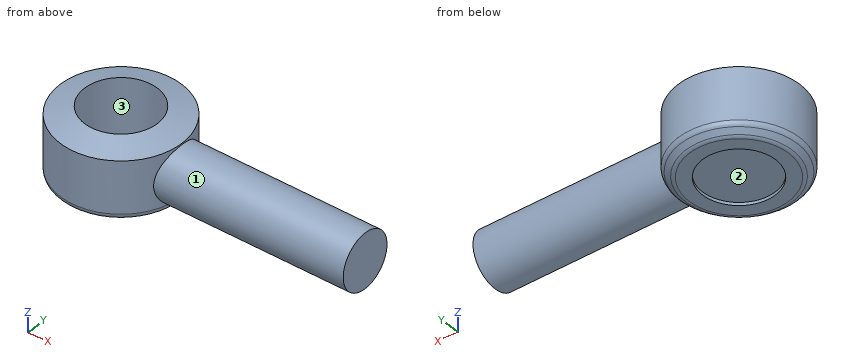
```python
from build123d import *

# Parameters (mm, degrees)
BOSS_EXTRUDE3_OUTLINE_W = 9
BOSS_EXTRUDE3_OUTLINE_H = 62.140537765


# Read off the part's stored shape, not the designer's step: Boss-Extrude3
with BuildPart() as part:
    # Sketch2 → Revolve1 (revolve)
    with BuildSketch(Plane(origin=(0, 0, 0), x_dir=(1, 0, 0), z_dir=(0, 1, 0)), mode=Mode.PRIVATE) as revolve1_sk:
        with BuildLine():
            Line((12, -12), (20, -9.430177972))
            Line((20, -9.430177972), (20, 7.708755689))
            ThreePointArc((20, 7.708755689), (19.794118127, 8.59257702), (19.218859855, 9.29443556))
            Line((19.218859855, 9.29443556), (17.53901118, 10.585679871))
            ThreePointArc((17.53901118, 10.585679871), (16.963828362, 10.893589151), (16.320151325, 11))
            Line((16.320151325, 11), (12, 11))
            Line((12, 11), (12, 10))
            Line((12, 10), (0, 10))
            Line((0, 10), (0, 7.49732498))
            Line((0, 7.49732498), (12, 7.49732498))
            Line((12, 7.49732498), (12, -12))
        make_face()
    revolve(revolve1_sk.sketch.rotate(Axis((0, 0, -10), (0, 0, 1)), 180), axis=Axis((0, 0, -10), (0, 0, 1)))

    # Boss-Extrude3 outline → Boss-Extrude3 (revolve)
    with BuildSketch(Plane.YX):
        with Locations((4.5, 48.929731117)):
            Rectangle(BOSS_EXTRUDE3_OUTLINE_W, BOSS_EXTRUDE3_OUTLINE_H)
    revolve(axis=Axis((0, 0, 0), (1, 0, 0)))


solid = part.part
```
Source: CAD feature listing. Evaluate the final solid. Frame: model axes, mm. Face numbers are marked on the shaded views. A direction names the side the tool comes from. Coordinates: 2 decimals unless noted, no trailing zeros. Order: outer loops, then holes, each group sorted by start corner. A loop starts at its lowest first (then second) coordinate and runs counter-clockwise, first axis right, second up. Notation, with made-up numbers: M 13,87 L 21,87 A9 ccw 21,94 Z; hole C -16.75,25 d6. An arc over 180 degrees is marked long. Write each question's results on one line, items separated by ' | '. Start each with the question number.
1) Line query: line 1 (Y direction, x = 0, z = 6.75); line 2 (Z direction, x = -4.5, y = -4); line 3 (Y direction, x = 0, z = -10.6). Output: solid intervals per line, ascending. Write a range as from..to.
2) Section query D-D (z = 5.75). Return the cut outline in (x, y), plus the area to 3 significant figures.
3) Section query C-C (y = 0). Return the cut outline in (x, z).
4) Section query B-B (x = 0). Return the cut outline in (y, z), plus the area to 3 significant figures.
5) Section query A-A (z = 0). Return the cut outline in (x, y), plus the area to 3 significant figures.
6) Access query for the marked faces 1, 2 and 3. Directions: +Z, -Z, +X, -X, +Y, -Y. A direction counts if a zero-diameter tool reaches every point of the face in a straight line with its end or side. Return the directions, or none.
7) Contact query for flat-ended pins moving along their axis: pin 1 Ø19 at (x, y) = (0, 0) entering from +Z; pin 2 Ø3 at (x, z) = (53.5, -2) entering from +Y; pin 3 Ø21.5 at (x, y) = (0, 0) entering from -Z; pin 4 Ø12 at (y, z) = (-9.5, -3.5) entering from +X. Output: stop coordinate, or through.
Answers:
1) line 1: y = -20..-12, 12..20 | line 2: z = -10..-7.5 | line 3: y = -17.52..-12, 12..17.52
2) outline: M 18.76,-6.92 L 80,-6.92 L 80,6.92 L 18.76,6.92 A20 ccw long Z; hole C 0,0 d24 | area: 1,640 mm^2
3) outline: M -20,-7.71 A2 ccw -19.22,-9.29 L -17.54,-10.59 A2 ccw -16.32,-11 L -12,-11 L -12,-10 L 12,-10 L 12,-11 L 16.32,-11 A2 ccw 17.54,-10.59 L 19.22,-9.29 A2 ccw 19.53,-9 L 80,-9 L 80,9 L 20,9 L 20,9.43 L 12,12 L 12,-7.5 L -12,-7.5 L -12,12 L -20,9.43 Z
4) outline: M -20,-7.71 A2 ccw -19.22,-9.29 L -17.54,-10.59 A2 ccw -16.32,-11 L -12,-11 L -12,-10 L 12,-10 L 12,-11 L 16.32,-11 A2 ccw 17.54,-10.59 L 19.22,-9.29 A2 ccw 20,-7.71 L 20,9.43 L 12,12 L 12,-7.5 L -12,-7.5 L -12,12 L -20,9.43 Z | area: 400 mm^2
5) outline: M 17.86,-9 L 80,-9 L 80,9 L 17.86,9 A20 ccw long Z; hole C 0,0 d24 | area: 1,900 mm^2
6) face 1: +X | face 2: -Z | face 3: +Z
7) pin 1: stops at z = -7.5 | pin 2: stops at y = 8.99 | pin 3: stops at z = -10 | pin 4: stops at x = 80
